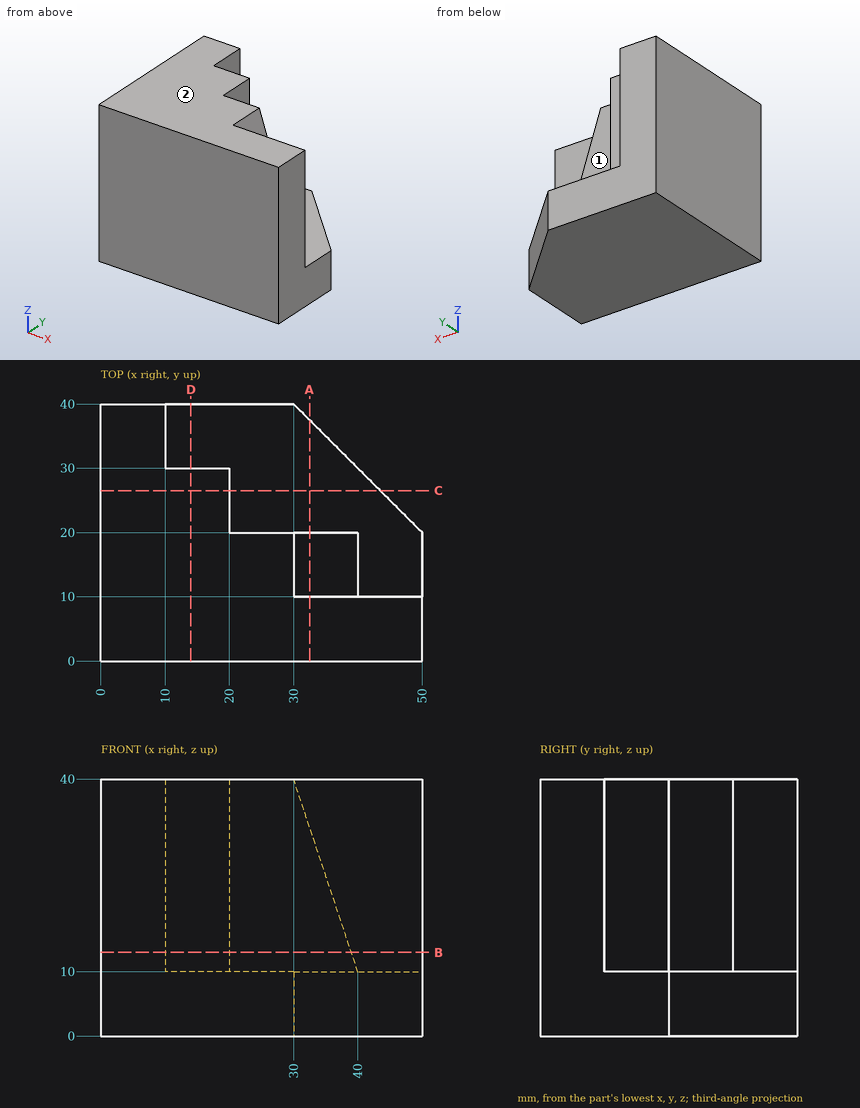
Check sheet for the drawn part. Datum: minimum x, y, z corner. Units: mm. A direction names the side the tool comes from. Round coordinates to 2 decimals unless told otherwise and drop trailing zeros. Write each loop counter-clockwise with the first axis right and the second up, starting at its lowest first coordinate (ties: lowest second). Pieces come first, ordered by that corner, then holes. Notation, with made-up numbers: (56.5, 4) - (63.5, 4) arc R16 cw to (63.5, 23) - close; hole circle Ø7 at (3, -32.5). An arc over 180 degrees is marked (long way). Write each question's results on one line, items separated by ' | '.
(1) Sectioned sample at A-A, the plane x = 32.5. Enter the section's corners in (y, z), plus the area to 3 significant figures.
Computed:
outline: (0, 0) - (37.5, 0) - (37.5, 10) - (20, 10) - (20, 32.5) - (10, 32.5) - (10, 40) - (0, 40) - close | area: 900 mm^2
(2) Sectioned sample at C-C, the plane y = 26.5. Enter the section's corners in (x, z), plus the area to 4 significant figures.
Computed:
outline: (0, 0) - (43.5, 0) - (43.5, 10) - (20, 10) - (20, 40) - (0, 40) - close | area: 1,035 mm^2
(3) Set-up check for the marked faces 1 and 2: record each of +Z, -Z, +X, -X, +Y, -Y from which the full face is reachable in a straight line by a thin tool's end or side.
Computed:
face 1: +Z, +X, +Y | face 2: +Z, +X, -X, +Y, -Y
(4) Sectioned sample at D-D, the plane x = 14. Enter the section's corners in (y, z).
Computed:
outline: (0, 0) - (40, 0) - (40, 10) - (30, 10) - (30, 40) - (0, 40) - close
(5) Thickness scan on probe 1 along X at (y, z) = (27, 18); probe 2 along Y at (x, z) = (17.5, 38.5). Record the ranges inside material, lowest first. Write a range as from..to.
Computed:
probe 1: x = 0..20 | probe 2: y = 0..30
(6) Sectioned sample at B-B, the plane z = 13. Enter the section's corners in (x, y).
Computed:
outline: (0, 0) - (50, 0) - (50, 10) - (39, 10) - (39, 20) - (20, 20) - (20, 30) - (10, 30) - (10, 40) - (0, 40) - close
(7) Depth check by flat-ended pin: pin 1 Ø22 at (x, z) = (25.5, 32.5) entering from +Y; pin 2 Ø3 at (y, z) = (36, 25) entering from +X; pin 3 Ø16 at (x, z) = (38, 26) entering from +Y. Enter the tip coordinate at first touch or a pass-through.
Computed:
pin 1: stops at y = 30 | pin 2: stops at x = 10 | pin 3: stops at y = 20
